Geometry: final body of the model. Coordinates: model frame, mm. Face numbers are marked on the shaded views. A direction names the side the tool comes from. Coordinates: 2 decimals unless noted, no trailing zeros. Write each loop counter-clockwise with the first axis right and the second up, starting at its lowest first coordinate (ties: lowest second). Pieces come first, ordered by that corner, then holes. Notation, with made-up numbers: (-27.5, 32.5) - (11.5, 32.5) arc R13 cw to (11.5, 38.5) - close; hole circle Ø10 at (55, 47). An arc over 180 degrees is marked (long way). Put each result on its own line as item: value.
```python
from build123d import *

# Parameters (mm, degrees)
SKETCH3_W           = 108
SKETCH3_H           = 152
BOSS_EXTRUDE1_DEPTH = 16
SKETCH7_W           = 98
SKETCH7_H           = 138
BOSS_EXTRUDE2_DEPTH = 4
SKETCH6_R           = 19.5
SKETCH6_RX          = 29.5
SKETCH6_RY          = 15
CUT_EXTRUDE2_DEPTH  = 16
SKETCH8_R           = 17
CUT_EXTRUDE3_DEPTH  = 10


with BuildPart() as part:
    # Sketch3 → Boss-Extrude1 (new body)
    with BuildSketch(Plane(origin=(0, 0, 0), x_dir=(1, 0, 0), z_dir=(0, 1, 0))):
        Rectangle(SKETCH3_W, SKETCH3_H)
    extrude(amount=BOSS_EXTRUDE1_DEPTH)

    # Sketch7 → Boss-Extrude2 (add)
    with BuildSketch(Plane.XZ):
        Rectangle(SKETCH7_W, SKETCH7_H)
    extrude(amount=BOSS_EXTRUDE2_DEPTH)

    # Sketch6 → Cut-Extrude2 (cut)
    with BuildSketch(Plane(origin=(0, 16, 0), x_dir=(1, 0, 0), z_dir=(0, 1, 0))):
        with Locations((22.271949374, 32)):
            Circle(SKETCH6_R)
        with Locations((22.271949374, -32)):
            Circle(SKETCH6_R)
        with Locations((-22.271949374, -32)):
            Circle(SKETCH6_R)
        with Locations((-22.271949374, 32)):
            Circle(SKETCH6_R)
        with Locations(Location((-22.271949374, 32), (0, 0, -90))):
            Ellipse(SKETCH6_RX, SKETCH6_RY)
        with Locations(Location((22.271949374, -32), (0, 0, -90))):
            Ellipse(SKETCH6_RX, SKETCH6_RY)
        with Locations(Location((-22.271949374, -32), (0, 0, -90))):
            Ellipse(SKETCH6_RX, SKETCH6_RY)
        with Locations(Location((22.271949374, 32), (0, 0, 90))):
            Ellipse(SKETCH6_RX, SKETCH6_RY)
    extrude(amount=-CUT_EXTRUDE2_DEPTH, mode=Mode.SUBTRACT)

    # Sketch8 → Cut-Extrude3 (cut)
    with BuildSketch(Plane(origin=(0, 0, 0), x_dir=(1, 0, 0), z_dir=(0, 1, 0))):
        with Locations(Location((-22.271949374, 32, 0), (0, 0, 270))):
            Circle(SKETCH8_R)
        with Locations(Location((22.271949374, 32, 0), (0, 0, 270))):
            Circle(SKETCH8_R)
        with Locations(Location((22.271949374, -32, 0), (0, 0, 270))):
            Circle(SKETCH8_R)
        with Locations(Location((-22.271949374, -32, 0), (0, 0, 270))):
            Circle(SKETCH8_R)
    extrude(amount=-CUT_EXTRUDE3_DEPTH, mode=Mode.SUBTRACT)


solid = part.part
```
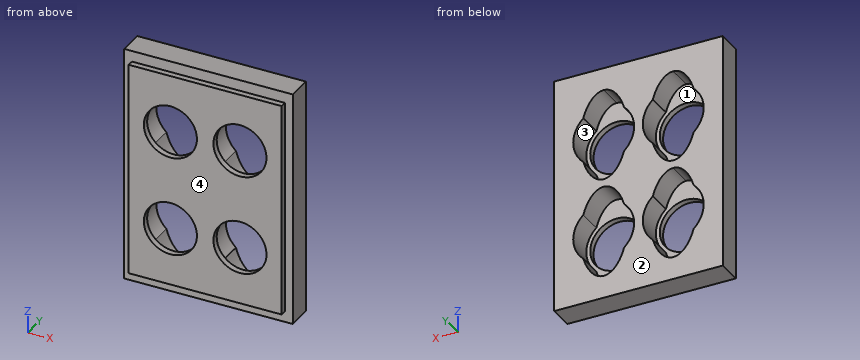
1. Ray query, probe 1 along X at (y, z) = (-3.1, 32); probe 2 along X at (y, z) = (-3, 45); probe 3 along Z at (x, y) = (-4.5, 6). Return the intervals inside material, ascending. Write a range as from..to.
Answer below:
probe 1: x = -49..-39.27, -5.27..5.27, 39.27..49
probe 2: x = -49..-33.23, -11.32..11.32, 33.23..49
probe 3: z = -76..-40.03, -23.97..23.97, 40.03..76
2. Section query D-D (y = 12.5). Count the separate pieces of the cut face and the enclosed holes in it, then the cut area to 3 significant figures.
Answer below:
separate pieces: 1
enclosed holes: 4
area: 10,100 mm²
3. Section query A-A (y = -2). Return loops of the section in (x, z), then the cut area to 3 significant figures.
Answer below:
outline: (-49, -69) - (49, -69) - (49, 69) - (-49, 69) - close; hole circle Ø34 at (-22.27, -32); hole circle Ø34 at (-22.27, 32); hole circle Ø34 at (22.27, -32); hole circle Ø34 at (22.27, 32)
area: 9,890 mm²
4. Section query C-C (z = -21). Return loops of the section in (x, y).
Answer below:
outline: (-54, 0) - (-49, 0) - (-49, -4) - (-35.23, -4) - (-35.23, 0) - (-38.37, 0) - (-38.37, 16) - (-54, 16) - close; (-9.31, -4) - (9.31, -4) - (9.31, 0) - (6.17, 0) - (6.17, 16) - (-6.17, 16) - (-6.17, 0) - (-9.31, 0) - close; (35.23, -4) - (49, -4) - (49, 0) - (54, 0) - (54, 16) - (38.37, 16) - (38.37, 0) - (35.23, 0) - close
5. Pin query (flat end, axial travel): pin 1 Ø6 at (x, z) = (10.5, 38.5) entering from +Y; pin 2 Ø4.5 at (x, y) = (-3.5, -2.5) entering from -Z; pin 3 Ø1.5 at (y, z) = (-1, 28.5) entering from -X; pin 4 Ø5 at (x, z) = (-35.5, -25.5) entering from +Y. Return the tip coordinate at first contact, or that it passes through.
Answer below:
pin 1: passes through
pin 2: stops at z = -69
pin 3: stops at x = -49
pin 4: stops at y = 0
6. Set-up query: the marked faces 3 and 4. Return all of +Z, -Z, +X, -X, +Y, -Y with unobstructed straight access to the full face (end or side cutting, diameter ignored); none if empty.
Answer below:
face 3: +Y
face 4: +Z, -Z, +X, -X, -Y
7. Mould query, pull axis Z, two halves, no side actions, for the marked faces 1 and 2. Classes: +Z half, -Z half, draft (parallel to the pull), parting line (faces both ways), or undercut.
Answer below:
face 1: undercut
face 2: draft
8. Section query B-B (z = 32). Return loops of the section in (x, y).
Answer below:
outline: (-54, 0) - (-49, 0) - (-49, -4) - (-39.27, -4) - (-39.27, 0) - (-41.77, 0) - (-41.77, 16) - (-54, 16) - close; (-5.27, -4) - (5.27, -4) - (5.27, 0) - (2.77, 0) - (2.77, 16) - (-2.77, 16) - (-2.77, 0) - (-5.27, 0) - close; (39.27, -4) - (49, -4) - (49, 0) - (54, 0) - (54, 16) - (41.77, 16) - (41.77, 0) - (39.27, 0) - close
